```python
from build123d import *

# Parameters (mm, degrees)
BOSS_EXTRUDE1_DEPTH      = 10
BOSS_EXTRUDE1_DEPTH_BACK = 5
BOSS_EXTRUDE2_DEPTH      = 5
CUT_EXTRUDE1_DEPTH       = 68.390151358
BOSS_EXTRUDE3_DEPTH      = 4
SKETCH7_R                = 1.75
BOSS_EXTRUDE4_DEPTH      = 2.4
SKETCH8_R                = 3.5
BOSS_EXTRUDE5_DEPTH      = 1
SKETCH9_R                = 5.1
SKETCH9_R_2              = 3.5
BOSS_EXTRUDE6_DEPTH      = 9


with BuildPart() as part:
    # Sketch2 → Boss-Extrude1 (new, two sides)
    with BuildSketch(Plane.XY.offset(12)) as boss_extrude1_sk:
        Polygon((-24.532899998, 27.1), (-33.204899998, 0), (-24.532899998, -27.1), (24.532899998, -27.1), (33.204899998, 0), (24.532899998, 27.1), align=None)
        Polygon((-23.36497619, 25.5), (-31.52497619, 0), (-23.36497619, -25.5), (23.36497619, -25.5), (31.52497619, 0), (23.36497619, 25.5), align=None, mode=Mode.SUBTRACT)
    extrude(amount=BOSS_EXTRUDE1_DEPTH)
    extrude(boss_extrude1_sk.sketch, amount=-BOSS_EXTRUDE1_DEPTH_BACK)

    # Sketch3 → Boss-Extrude2 (add)
    with BuildSketch(Plane.XY.offset(22)):
        Polygon((29.75, 16.1), (59.85, 16.1), (59.85, -16.1), (29.75, -16.1), (28.052899998, -16.1), (28.564899998, -14.5), (29.75, -14.5), (58.25, -14.5), (58.25, 14.5), (29.75, 14.5), (28.564899998, 14.5), (28.052899998, 16.1), align=None)
    extrude(amount=-BOSS_EXTRUDE2_DEPTH)

    # Sketch4 → Cut-Extrude1 (cut, through all)
    with BuildSketch(Plane(origin=(0, 0, 7), x_dir=(-1, 0, 0), z_dir=(0, 0, -1))):
        Polygon((-26.88497619, 14.5), (-28.564899998, 14.5), (-33.204899998, 0), (-28.564899998, -14.5), (-26.88497619, -14.5), (-31.52497619, 0), align=None)
    extrude(amount=-CUT_EXTRUDE1_DEPTH, mode=Mode.SUBTRACT)

    # Sketch5 → Boss-Extrude3 (add)
    with BuildSketch(Plane.XY.offset(22)):
        Polygon((29.25, 4.3), (29.25, 14), (29.25, 14.5), (27.65, 14.5), (27.65, 14), (27.65, 5.9), (-4.35, 5.9), (-4.35, -5.9), (27.65, -5.9), (27.65, -14), (27.65, -14.5), (29.25, -14.5), (29.25, -14), (29.25, -4.3), (-2.75, -4.3), (-2.75, 4.3), align=None)
    extrude(amount=-BOSS_EXTRUDE3_DEPTH)

    # Sketch7 → Boss-Extrude4 (add)
    with BuildSketch(Plane.XY.offset(22)):
        Polygon((37.25, 12.1), (37.25, 14.5), (29.25, 14.5), (29.25, 4.3), (5.85, 4.3), (5.85, -4.3), (29.25, -4.3), (29.25, -14.5), (58.25, -14.5), (58.25, -11.6), (31.65, -11.6), (31.65, 12.1), align=None)
        with Locations((23.75, 0)):
            Circle(SKETCH7_R, mode=Mode.SUBTRACT)
    extrude(amount=-BOSS_EXTRUDE4_DEPTH)

    # Sketch8 → Boss-Extrude5 (add)
    with BuildSketch(Plane.XY.offset(22)):
        Polygon((27.65, -5.9), (27.65, -14.5), (26.88497619, -14.5), (23.36497619, -25.5), (-23.36497619, -25.5), (-31.52497619, 0), (-23.36497619, 25.5), (23.36497619, 25.5), (26.88497619, 14.5), (27.65, 14.5), (27.65, 5.9), (-4.35, 5.9), (-4.35, -5.9), align=None)
        with Locations((-18.25, 18.25)):
            Circle(SKETCH8_R, mode=Mode.SUBTRACT)
        with Locations((18.25, 18.25)):
            Circle(SKETCH8_R, mode=Mode.SUBTRACT)
        with Locations((18.25, -18.25)):
            Circle(SKETCH8_R, mode=Mode.SUBTRACT)
        with Locations((-18.25, -18.25)):
            Circle(SKETCH8_R, mode=Mode.SUBTRACT)
    extrude(amount=-BOSS_EXTRUDE5_DEPTH)

    # Sketch9 → Boss-Extrude6 (add)
    with BuildSketch(Plane(origin=(0, 0, 21), x_dir=(-1, 0, 0), z_dir=(0, 0, -1))):
        with Locations(Location((-18.25, 18.25, 0), (0, 0, 180))):
            Circle(SKETCH9_R)
        with Locations(Location((-18.25, 18.25, 0), (0, 0, 180))):
            Circle(SKETCH9_R_2, mode=Mode.SUBTRACT)
        with Locations(Location((18.25, 18.25, 0), (0, 0, 180))):
            Circle(SKETCH9_R)
        with Locations(Location((18.25, 18.25, 0), (0, 0, 180))):
            Circle(SKETCH9_R_2, mode=Mode.SUBTRACT)
        with Locations(Location((18.25, -18.25, 0), (0, 0, 180))):
            Circle(SKETCH9_R)
        with Locations(Location((18.25, -18.25, 0), (0, 0, 180))):
            Circle(SKETCH9_R_2, mode=Mode.SUBTRACT)
        with Locations(Location((-18.25, -18.25, 0), (0, 0, 180))):
            Circle(SKETCH9_R)
        with Locations(Location((-18.25, -18.25, 0), (0, 0, 180))):
            Circle(SKETCH9_R_2, mode=Mode.SUBTRACT)
    extrude(amount=BOSS_EXTRUDE6_DEPTH)


solid = part.part
```
Work out the finished part from the listing and answer in its coordinate system (mm). A direction names the side the tool comes from. Give positions to 0.01 mm unless a question says otherwise; leave off trailing zeros. Loops run counter-clockwise (first coordinate to the right, second up) from the corner with the lowest first, then second, coordinate; pieces in that order, holes last. Notation, with made-up numbers: (26.5, 83.25) -> (41.5, 83.25) arc R26 cw to (41.5, 119.25) -> close; hole circle Ø9 at (41.25, 6.25). An arc over 180 degrees is marked (long way). Put each result on its own line as item: value. Start each with the question number.
Item 1: The part is cut by section B-B (z = 8.25). Give the vertices of the cut face in (x, y), then the cut area to 3 significant figures.
Item 2: Each of these flat-tipped pins is pushed along its axis until it touches: P1, Ø1.2, axis at x = 35, z = 20.5, coming from the -Y side; P2, Ø14.5, axis at x = 25.5, y = -1, coming from the -Z side; P3, Ø1.5, axis at x = 46.5, z = 19, coming from the +Y side. Where does it stop, or does it pass through?
Item 3: The part is cut by section A-A (x = -18.25). Give the vertices of the cut face in (y, z).
Item 4: The part is cut by section D-D (x = 10). Give the vertices of the cut face in (y, z), then the cut area to 3 significant figures.
Item 5: The mould has two halves that part along Y. Classify faces 1 (the face through (26.52, -20.89, 14.6)), 2 (the face through (-30, 6, 7)), 3 (the face through (26.577, 20.712, 14.605)), 4 (the face through (41, -14.5, 18)): released by +Y, released by -Y, zero draft, split by the parting line, or undercut.
Item 6: The part is cut by section C-C (y = -18.25). Give the vertices of the cut face in (x, z).
Item 7: Which of the six approach directions +Z, -Z, +X, -X, +Y, -Y give full straight-line access (tool end or side, diameter ignored) to faces 5 (the face through (44, -16.1, 20)), 6 (the face through (5.85, 0, 21)), 7 (the face through (27.65, 10, 20)), 8 (the face through (-28.81, 13.74, 14.6))?
Item 8: Find the intervals of material crossed by L1, parallel to Y at x = 18.25, z = 15.5; L2, parallel to Y at x = 18.25, z = 21.85; L3, parallel to Y at x = 23.75, z = 21.45, in increasing order. Write a range as [from, to].
Answers below:
1. outline: (-33.2, 0) -> (-24.53, -27.1) -> (24.53, -27.1) -> (28.56, -14.5) -> (26.88, -14.5) -> (23.36, -25.5) -> (-23.36, -25.5) -> (-31.52, 0) -> (-23.36, 25.5) -> (23.36, 25.5) -> (26.88, 14.5) -> (28.56, 14.5) -> (24.53, 27.1) -> (-24.53, 27.1) -> close
1. area: 281 mm2
2. P1: y = -16.1
2. P2: z = 18
2. P3: y = 16.1
3. outline: (-27.1, 7) -> (-25.5, 7) -> (-25.5, 21) -> (-23.35, 21) -> (-23.35, 12) -> (-21.75, 12) -> (-21.75, 22) -> (-27.1, 22) -> close; (-14.75, 12) -> (-13.15, 12) -> (-13.15, 21) -> (13.15, 21) -> (13.15, 12) -> (14.75, 12) -> (14.75, 22) -> (-14.75, 22) -> close; (21.75, 12) -> (23.35, 12) -> (23.35, 21) -> (25.5, 21) -> (25.5, 7) -> (27.1, 7) -> (27.1, 22) -> (21.75, 22) -> close
4. outline: (-27.1, 7) -> (-25.5, 7) -> (-25.5, 21) -> (-5.9, 21) -> (-5.9, 18) -> (-4.3, 18) -> (-4.3, 19.6) -> (4.3, 19.6) -> (4.3, 18) -> (5.9, 18) -> (5.9, 21) -> (25.5, 21) -> (25.5, 7) -> (27.1, 7) -> (27.1, 22) -> (-27.1, 22) -> close
4. area: 121 mm2
5. face 1: released by -Y
5. face 2: zero draft
5. face 3: released by +Y
5. face 4: undercut
6. outline: (-27.36, 7) -> (-25.68, 7) -> (-25.68, 21) -> (-23.35, 21) -> (-23.35, 12) -> (-21.75, 12) -> (-21.75, 22) -> (-27.36, 22) -> close; (-14.75, 12) -> (-13.15, 12) -> (-13.15, 21) -> (13.15, 21) -> (13.15, 12) -> (14.75, 12) -> (14.75, 22) -> (-14.75, 22) -> close; (21.75, 12) -> (23.35, 12) -> (23.35, 21) -> (25.68, 21) -> (25.68, 7) -> (27.36, 7) -> (27.36, 22) -> (21.75, 22) -> close
7. face 5: +Z, -Z, +X, -Y
7. face 6: +Z, -Z
7. face 7: -Z
7. face 8: +Z, -Z, -X, +Y
8. L1: [-27.1, -25.5], [-23.35, -21.75], [-14.75, -13.15], [13.15, 14.75], [21.75, 23.35], [25.5, 27.1]
8. L2: [-27.1, -21.75], [-14.75, 14.75], [21.75, 27.1]
8. L3: [-27.1, -1.75], [1.75, 27.1]
